Verification items for the finished model (mm, model axes). Face numbers are marked on the shaded views. A direction names the side the tool comes from. Coordinates: 2 decimals unless noted, no trailing zeros. Loops run counter-clockwise (first coordinate to the right, second up) from the corner with the lowest first, then second, coordinate; pieces in that order, holes last. Notation, with made-up numbers: (-4.5, -8) - (29.5, -8) arc R20 ccw to (29.5, -1) - close; hole circle Ø7 at (89, 22). An arc over 180 degrees is marked (long way). Answer as CSV lines item,"result". Start each with the question number.
1. Material ranges on line 1 (Y direction, x = 0, z = -3.45); line 2 (Z direction, x = -9.5, y = 0.75); line 3 (Z direction, x = -0.5, y = -3), recorded low to high. Write a range as [from, to].
2. Cross-section at B-B (x = 12). Enter the section's corners in (y, z), plus the area to 3 significant figures.
3. Cross-section at C-C (y = 0). Enter the section's corners in (x, z), plus the area to 3 significant figures.
4. Release check for a two-part mould opening along X. For the marked faces 1, 2, 3 and 4 record: pulls with the +X half, pulls with the -X half, needs draft (parallel to the pull), parting line crosses it, or undercut.
5. Cross-section at D-D (x = 8). Enter the section's corners in (y, z), plus the area to 3 significant figures.
6. Set-up check for the marked faces 5, 6 and 7: record each of +Z, -Z, +X, -X, +Y, -Y from which the full face is reachable in a straight line by a thin tool's end or side.
7. Cross-section at A-A (y = 13). Enter the section's corners in (x, z), plus the area to 3 significant figures.
8. Gauge pin test, flat ends, axial feed: P1, Ø7, axis at x = 12.5, y = -6, coming from the -Z side; P2, Ø2, axis at x = 6, y = 7.5, coming from the -Z side; P3, Ø5, axis at y = -7.5, z = -19, coming from the -X side; P4, Ø8, axis at x = 0.5, y = -3.5, coming from the +Z side. Record the tip position at first contact, or that the pin passes through.
```python
from build123d import *

# Parameters (mm, degrees)
HOLE_WIZARD_M4_1_D  = 3.3
SKETCH_4_OUTSIDE_W  = 44.75
SKETCH_4_OUTSIDE_H  = 44.75
CUT_EXTRUDE_4_DEPTH = 3
CHAMFER_1_SIZE      = 1


with BuildPart() as part:
    # 草图1 → 旋转1 (revolve)
    with BuildSketch(Plane(origin=(0, 0, 0), x_dir=(0, 0, -1), z_dir=(1, 0, 0)), mode=Mode.PRIVATE) as revolve_1_sk:
        Polygon((0, 0), (29, 0), (29, 3), (19, 3), (19, 10), (18, 10), (18, 8.5), (17, 8.5), (17, 10), (9, 10), (9, 10.5), (5, 10.5), (5, 16), (2, 16), (2, 7.5), (0, 7.5), align=None)
    revolve(revolve_1_sk.sketch.rotate(Axis((0, 0, 0), (0, 0, -1)), 180), axis=Axis((0, 0, 0), (0, 0, -1)))

    # M4 螺纹孔1 (through all)
    with Locations(Plane.XY.offset(-2)):
        with Locations((0, 13), (11.258330249, -6.5), (-11.258330249, -6.5)):
            Hole(HOLE_WIZARD_M4_1_D / 2)

    # 草图4 outside → 切除-拉伸4 (cut)
    with BuildSketch(Plane.XY.offset(-2)):
        Rectangle(SKETCH_4_OUTSIDE_W, SKETCH_4_OUTSIDE_H)
        with BuildLine():
            Line((4, 15.491933385), (4, 9.708243919))
            ThreePointArc((4, 9.708243919), (9.09326674, 5.25), (10.40758586, -1.390020345))
            Line((10.40758586, -1.390020345), (15.416407865, -4.281865077))
            ThreePointArc((15.416407865, -4.281865077), (13.856406461, -8), (11.416407865, -11.210068308))
            Line((11.416407865, -11.210068308), (6.40758586, -8.318223575))
            ThreePointArc((6.40758586, -8.318223575), (0, -10.5), (-6.40758586, -8.318223575))
            Line((-6.40758586, -8.318223575), (-11.416407865, -11.210068308))
            ThreePointArc((-11.416407865, -11.210068308), (-13.856406461, -8), (-15.416407865, -4.281865077))
            Line((-15.416407865, -4.281865077), (-10.40758586, -1.390020345))
            ThreePointArc((-10.40758586, -1.390020345), (-9.09326674, 5.25), (-4, 9.708243919))
            Line((-4, 9.708243919), (-4, 15.491933385))
            ThreePointArc((-4, 15.491933385), (0, 16), (4, 15.491933385))
        make_face(mode=Mode.SUBTRACT)
    extrude(amount=-CUT_EXTRUDE_4_DEPTH, mode=Mode.SUBTRACT)

    # 倒角1
    chamfer_1_edges = [part.edges().sort_by_distance(p)[0] for p in [
        (0, 7.5, 0),
    ]]
    chamfer(chamfer_1_edges, length=CHAMFER_1_SIZE)


solid = part.part
```
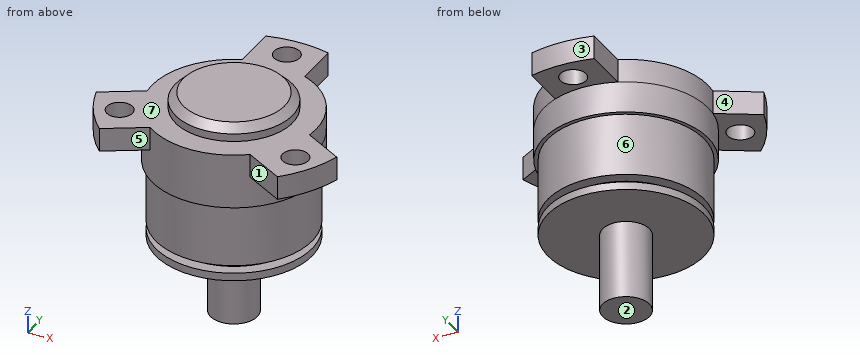
Values follow:
1,line 1,"y = [-10.5, 11.35], [14.65, 16]"
1,line 2,"z = [-19, -18], [-17, -2]"
1,line 3,"z = [-19, 0]"
2,outline,"(-10.58, -5) - (-7.97, -5) - (-7.97, -2) - (-10.58, -2) - close; (-5.03, -5) - (-2.31, -5) - (-2.31, -2) - (-5.03, -2) - close"
2,area,"16.0 mm²"
3,outline,"(-10.5, -9) - (-10, -9) - (-10, -17) - (-8.5, -17) - (-8.5, -18) - (-10, -18) - (-10, -19) - (-3, -19) - (-3, -29) - (3, -29) - (3, -19) - (10, -19) - (10, -18) - (8.5, -18) - (8.5, -17) - (10, -17) - (10, -9) - (10.5, -9) - (10.5, -2) - (7.5, -2) - (7.5, -1) - (6.5, 0) - (-6.5, 0) - (-7.5, -1) - (-7.5, -2) - (-10.5, -2) - close"
3,area,"433 mm²"
4,face 1,"undercut"
4,face 2,"needs draft"
4,face 3,"parting line crosses it"
4,face 4,"pulls with the -X half"
5,outline,"(-9.24, -5) - (-6.8, -5) - (-6.8, -9) - (-6, -9) - (-6, -17) - (-2.87, -17) - (-2.87, -18) - (-6, -18) - (-6, -19) - (6, -19) - (6, -18) - (2.87, -18) - (2.87, -17) - (6, -17) - (6, -9) - (6.8, -9) - (6.8, -2) - (-9.24, -2) - close"
5,area,"216 mm²"
6,face 5,"+Z, -Z, -Y"
6,face 6,"-Z"
6,face 7,"+Z"
7,outline,"(-4, -5) - (-1.65, -5) - (-1.65, -2) - (-4, -2) - close; (1.65, -5) - (4, -5) - (4, -2) - (1.65, -2) - close"
7,area,"14.1 mm²"
8,P1,"stops at z = -9"
8,P2,"stops at z = -19"
8,P3,"stops at x = -8.66"
8,P4,"stops at z = 0"
